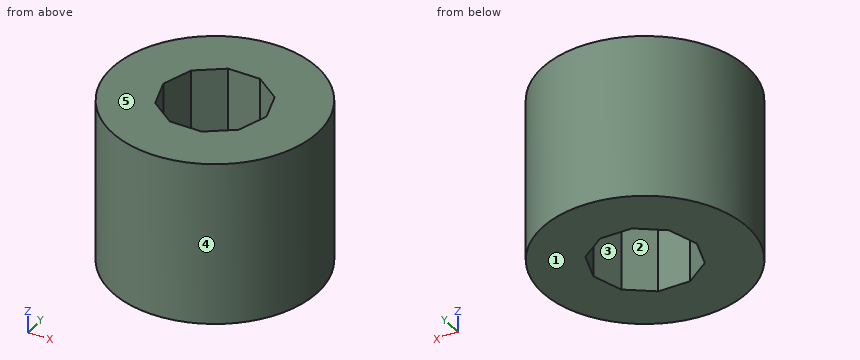
from build123d import *

# Parameters (mm, degrees)
F0_R     = 55.837677
F1_DEPTH = 88.646
F3_DEPTH = 88.647


with BuildPart() as f1:
    # F0 (on Top) → F1 (new body)
    with BuildSketch(Plane.XY):
        Circle(F0_R)
    extrude(amount=F1_DEPTH)

    # F2 (on Top) → F3 (cut, through all)
    with BuildSketch(Plane.XY):
        Polygon((8.678742, 26.710423), (-8.678742, 26.710423), (-22.721243, 16.507949), (-28.085, 0), (-22.721243, -16.507949), (-8.678742, -26.710423), (8.678742, -26.710423), (22.721243, -16.507949), (28.085, 0), (22.721243, 16.507949), align=None)
    extrude(amount=F3_DEPTH, mode=Mode.SUBTRACT)


solid = f1.part
Model file for the job. Use its own axes, mm. Face numbers are marked on the shaded views. A direction names the side the tool comes from. Give positions to 0.01 mm unless a question says otherwise; leave off trailing zeros. Write each loop counter-clockwise with the first axis right and the second up, starting at its lowest first coordinate (ties: lowest second). Pieces come first, ordered by that corner, then holes. Notation, with made-up numbers: (-13, 21.25) -> (3, 21.25) arc R16 cw to (3, 30.25) -> close; hole circle Ø8 at (29.25, 18). An arc over 180 degrees is marked (long way). Write item = value, one per line.
(1) Slice it at D-D, the plane y = 31. Give the cut face in (x, z), then the cut area to 3 significant figures.
Determined:
outline = (-46.44, 0) -> (46.44, 0) -> (46.44, 88.65) -> (-46.44, 88.65) -> close
area = 8,230 mm2
(2) Slice it at A-A, the plane z = 30. Give the cut face in (x, y) (3 decimals).
Determined:
outline = circle Ø111.675 at (0, 0); hole (-28.085, 0) -> (-22.721, -16.508) -> (-8.679, -26.71) -> (8.679, -26.71) -> (22.721, -16.508) -> (28.085, 0) -> (22.721, 16.508) -> (8.679, 26.71) -> (-8.679, 26.71) -> (-22.721, 16.508) -> close
(3) Tool access for the marked faces 1 and 2: list every direction of +Z, -Z, +X, -X, +Y, -Y with a clear straight run to the whole face (end or side of a thin tool).
Determined:
face_1 = -Z, +X, -X, +Y, -Y
face_2 = +Z, -Z
(4) Slice it at C-C, the plane y = -23.5. Give the cut face in (x, z).
Determined:
outline = (-50.65, 0) -> (-13.1, 0) -> (-13.1, 88.65) -> (-50.65, 88.65) -> close; (13.1, 0) -> (50.65, 0) -> (50.65, 88.65) -> (13.1, 88.65) -> close
(5) Mould opens along Y. For the marked faces 3, 4 and 5 say: released by +Y, released by -Y, zero draft, split by the parting line, or undercut.
Determined:
face_3 = undercut
face_4 = split by the parting line
face_5 = zero draft
(6) Slice it at B-B, the plane x = 20.5. Give the cut face in (y, z), then the cut area to 3 significant figures.
Determined:
outline = (-51.94, 0) -> (-18.12, 0) -> (-18.12, 88.65) -> (-51.94, 88.65) -> close; (18.12, 0) -> (51.94, 0) -> (51.94, 88.65) -> (18.12, 88.65) -> close
area = 6,000 mm2
(7) Probe line 1 along X through (y, z) = (-16.5, 42.5); line 2 along Y through (x, z) = (13.5, 12.5); line 3 along X through (y, z) = (2.5, 37). List the from-to ranges inside material, lowest first.
Determined:
line_1 = -53.34 to -22.72, 22.72 to 53.34
line_2 = -54.18 to -23.21, 23.21 to 54.18
line_3 = -55.78 to -27.27, 27.27 to 55.78
(8) Flat gauge pins, fed straight in: P1, Ø3, axis at y = -15.5, z = 57.5, coming from the +X side; P2, Ø5, axis at y = -8, z = 48, coming from the -X side; P3, Ø1.5, axis at y = -29, z = 76, coming from the -X side. Where does each tip first touch, or does it go through?
Determined:
P1 = 54.05
P2 = -55.57
P3 = -48.16
